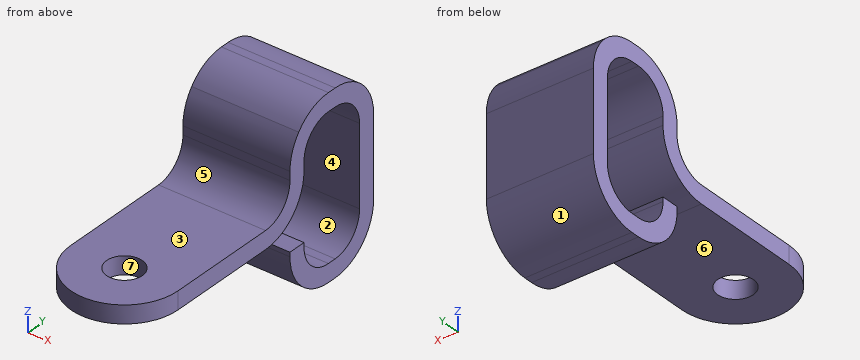
from build123d import *

# Parameters (mm, degrees)
EXTRUDE_1_DEPTH     = 1
SKETCH_2_R          = 1
CUT_EXTRUDE_1_DEPTH = 28.116287625
OTHER_START         = -3
OTHER_1_DEPTH       = 6
OTHER_1_2_DEPTH     = 6
OTHER_2_DEPTH       = 6
OTHER_2_2_DEPTH     = 6
OTHER_START_2       = -5.911973487
OTHER_2_3_OUTLINE_W = 6
OTHER_2_3_OUTLINE_H = 4
OTHER_2_3_DEPTH     = 12.911973487
OTHER_START_3       = -10.873389715
OTHER_2_4_OUTLINE_R = 1
OTHER_2_4_DEPTH     = 1
OTHER_START_4       = -8.133389715
OTHER_2_5_OUTLINE_W = 6
OTHER_2_5_OUTLINE_H = 1
OTHER_2_5_DEPTH     = 0.481416228
OTHER_2_6_DEPTH     = 6
OTHER_2_7_DEPTH     = 6


with BuildPart() as part:
    # Sketch 1 → Бобышка-Вытянуть1 (new body)
    with BuildSketch(Plane(origin=(0, 0, 0), x_dir=(1, 0, 0), z_dir=(0, 1, 0))):
        with BuildLine():
            Line((-3, 26.931265373), (-3, -3.068734627))
            ThreePointArc((-3, -3.068734627), (0, -6.068734627), (3, -3.068734627))
            Line((3, -3.068734627), (3, 26.931265373))
            Line((3, 26.931265373), (-3, 26.931265373))
        make_face()
    extrude(amount=EXTRUDE_1_DEPTH)

    # Sketch 2 → Вырез-Вытянуть1 (cut, through all)
    with BuildSketch(Plane(origin=(0, 1, 0), x_dir=(1, 0, 0), z_dir=(0, 1, 0))):
        with Locations(Location((0, -3.068734627, 0), (0, 0, 270))):
            Circle(SKETCH_2_R)
    extrude(amount=-CUT_EXTRUDE_1_DEPTH, mode=Mode.SUBTRACT)

    # Other 1: read off the stored shape, not the designer's step
    # Other 1 outline → Other 1 (cut)
    with BuildSketch(Plane.YZ.offset(OTHER_START)):
        with BuildLine():
            Line((1, -26.931265373), (1, -5.288574535))
            ThreePointArc((1, -5.288574535), (0.26258199, -4.342443478), (0, -3.171973487))
            Line((0, -3.171973487), (0, -26.931265373))
            Line((0, -26.931265373), (1, -26.931265373))
        make_face()
    extrude(amount=OTHER_1_DEPTH, mode=Mode.SUBTRACT)

    # Other 1 2 outline → Other 1 2 (add)
    with BuildSketch(Plane.YZ.offset(OTHER_START)):
        with BuildLine():
            Line((2.74, -5.911973487), (22.980708114, -5.911973487))
            Line((22.980708114, -5.911973487), (22.980708114, -4.911973487))
            Line((22.980708114, -4.911973487), (2.74, -4.911973487))
            ThreePointArc((2.74, -4.911973487), (1.509634201, -4.402339286), (1, -3.171973487))
            Line((1, -3.171973487), (1, -5.288574535))
            ThreePointArc((1, -5.288574535), (1.815848193, -5.75141983), (2.74, -5.911973487))
        make_face()
    extrude(amount=OTHER_1_2_DEPTH)

    # Other 2: read off the stored shape, not the designer's step
    # Other 2 outline → Other 2 (cut)
    with BuildSketch(Plane.YZ.offset(OTHER_START)):
        with BuildLine():
            ThreePointArc((7.221416228, -4.911973487), (8.391886219, -5.174555476), (9.338017277, -5.911973487))
            Line((9.338017277, -5.911973487), (22.980708114, -5.911973487))
            Line((22.980708114, -5.911973487), (22.980708114, -4.911973487))
            Line((22.980708114, -4.911973487), (7.221416228, -4.911973487))
        make_face()
    extrude(amount=OTHER_2_DEPTH, mode=Mode.SUBTRACT)

    # Other 2 2 outline → Other 2 2 (add)
    with BuildSketch(Plane.YZ.offset(OTHER_START)):
        with BuildLine():
            Line((8.961416228, -7.651973487), (8.961416228, -12.133389715))
            ThreePointArc((8.961416228, -12.133389715), (8.451782027, -13.363755514), (7.221416228, -13.873389715))
            Line((7.221416228, -13.873389715), (6.74, -13.873389715))
            ThreePointArc((6.74, -13.873389715), (5.509634201, -13.363755514), (5, -12.133389715))
            Line((5, -12.133389715), (5, -11.892681601))
            Line((5, -11.892681601), (4, -11.892681601))
            Line((4, -11.892681601), (4, -12.133389715))
            ThreePointArc((4, -12.133389715), (4.80252742, -14.070862295), (6.74, -14.873389715))
            Line((6.74, -14.873389715), (7.221416228, -14.873389715))
            ThreePointArc((7.221416228, -14.873389715), (9.158888808, -14.070862295), (9.961416228, -12.133389715))
            Line((9.961416228, -12.133389715), (9.961416228, -7.651973487))
            ThreePointArc((9.961416228, -7.651973487), (9.800862571, -6.72782168), (9.338017277, -5.911973487))
            Line((9.338017277, -5.911973487), (7.221416228, -5.911973487))
            ThreePointArc((7.221416228, -5.911973487), (8.451782028, -6.421607687), (8.961416228, -7.651973487))
        make_face()
    extrude(amount=OTHER_2_2_DEPTH)

    # Other 2 3 outline → Other 2 3 (cut)
    with BuildSketch(Plane.XY.offset(OTHER_START_2)):
        with Locations((0, 2)):
            Rectangle(OTHER_2_3_OUTLINE_W, OTHER_2_3_OUTLINE_H)
    extrude(amount=OTHER_2_3_DEPTH, mode=Mode.SUBTRACT)

    # Other 2 6 outline → Other 2 6 (cut)
    with BuildSketch(Plane.YZ.offset(OTHER_START)):
        with BuildLine():
            ThreePointArc((4.623398951, -5.911973487), (5.569530009, -5.174555476), (6.74, -4.911973487))
            Line((6.74, -4.911973487), (4, -4.911973487))
            Line((4, -4.911973487), (4, -5.911973487))
            Line((4, -5.911973487), (4.623398951, -5.911973487))
        make_face()
    extrude(amount=OTHER_2_6_DEPTH, mode=Mode.SUBTRACT)



with BuildPart() as body_2:
    # Other 2 4 outline → Other 2 4 (new body)
    with BuildSketch(Plane.XY.offset(OTHER_START_3)):
        with BuildLine():
            Line((3, 1), (-3, 1))
            Line((-3, 1), (-3, -3.980708114))
            ThreePointArc((-3, -3.980708114), (0, -6.980708114), (3, -3.980708114))
            Line((3, -3.980708114), (3, 1))
        make_face()
        with Locations((0, -3.980708114)):
            Circle(OTHER_2_4_OUTLINE_R, mode=Mode.SUBTRACT)
    extrude(amount=OTHER_2_4_DEPTH)


with BuildPart() as body_3:
    # Other 2 5 outline → Other 2 5 (new body)
    with BuildSketch(Plane.XY.offset(OTHER_START_4)):
        with Locations((0, 4.5)):
            Rectangle(OTHER_2_5_OUTLINE_W, OTHER_2_5_OUTLINE_H)
    extrude(amount=OTHER_2_5_DEPTH)


with BuildPart() as part_1:
    add(part.part)

    add(body_2.part)  # Other 2 7 merges body 2

    add(body_3.part)  # Other 2 7 merges body 3
    # Other 2 7 outline → Other 2 7 (add)
    with BuildSketch(Plane.YZ.offset(OTHER_START)):
        with BuildLine():
            Line((6.74, -5.911973487), (4.623398951, -5.911973487))
            ThreePointArc((4.623398951, -5.911973487), (4.160553657, -6.72782168), (4, -7.651973487))
            Line((4, -7.651973487), (5, -7.651973487))
            ThreePointArc((5, -7.651973487), (5.5096342, -6.421607687), (6.74, -5.911973487))
        make_face()
        with BuildLine():
            Line((1, -10.873389715), (2.26, -10.873389715))
            ThreePointArc((2.26, -10.873389715), (4.19747258, -10.070862295), (5, -8.133389715))
            Line((5, -8.133389715), (4, -8.133389715))
            ThreePointArc((4, -8.133389715), (3.490365799, -9.363755514), (2.26, -9.873389715))
            Line((2.26, -9.873389715), (1, -9.873389715))
            Line((1, -9.873389715), (1, -10.873389715))
        make_face()
    extrude(amount=OTHER_2_7_DEPTH)


solid = part_1.part
Geometry check sheet. Reference: the model listing, model coordinates, mm. Face numbers are marked on the shaded views. A direction names the side the tool comes from. Round coordinates to 2 decimals unless told otherwise and drop trailing zeros. Loops run counter-clockwise (first coordinate to the right, second up) from the corner with the lowest first, then second, coordinate; pieces in that order, holes last.
Item 1: Cross-section at C-C on z = -13. Record the boundary of the cut face in (x, y), then the cut area to 3 significant figures.
Item 2: Cross-section at B-B on y = -4.75. Record the boundary of the cut face in (x, z).
Item 3: Thickness scan on line 1 (Z direction, x = 0.65, y = 6.75); line 2 (Y direction, x = -1.4, z = -12.25); line 3 (Y direction, x = 0, z = -10.4). Record the ranges inside material, lowest first.
Item 4: Gauge pin test, flat ends, axial feed: pin 1 (2.5 mm diameter, centred on x = 0, y = -3.98, fed in from +Z); pin 2 (0.5 mm diameter, centred on x = 0.5, y = 4.5, fed in from +Z); pin 3 (0.5 mm diameter, centred on x = -1, z = -8, fed in from -Y). Record the tip position at first contact, or that the pin passes through.
Item 5: Access from +Z, -Z, +X, -X, +Y, -Y to the whole of each face (thin tool, end or side, straight path). Record for the marked faces 1, 2 and 3.
Item 6: Cross-section at D-D on x = -1.7. Record the boundary of the cut face in (y, z).
Item 7: Mould release check, pull along Z, two halves, no side actions. Record for the marked faces 4, 5, 6 and 7: pulls with the +Z half, pulls with the -Z half, needs draft (parallel to the pull), parting line crosses it, or undercut.
Item 8: Cross-section at A-A on x = 0. Record the boundary of the cut face in (y, z).
Answer sheet:
1. outline: (-3, 4.14) - (3, 4.14) - (3, 5.23) - (-3, 5.23) - close; (-3, 8.73) - (3, 8.73) - (3, 9.82) - (-3, 9.82) - close
1. area: 13.1 mm2
2. outline: (-2.9, -10.87) - (-0.64, -10.87) - (-0.64, -9.87) - (-2.9, -9.87) - close; (0.64, -10.87) - (2.9, -10.87) - (2.9, -9.87) - (0.64, -9.87) - close
3. line 1: z = -14.87 to -13.87, -5.91 to -4.91
3. line 2: y = 4 to 5, 8.96 to 9.96
3. line 3: y = -6.98 to -4.98, -2.98 to 3.8, 8.96 to 9.96
4. pin 1: stops at z = -9.87
4. pin 2: stops at z = -5.77
4. pin 3: stops at y = 4
5. face 1: -Z, +X, -X, +Y
5. face 2: +X, -X
5. face 3: +Z, +X, -X, -Y
6. outline: (-6.45, -10.87) - (2.26, -10.87) arc R2.74 ccw to (5, -8.13) - (5, -7.65) arc R1.74 cw to (6.74, -5.91) - (7.22, -5.91) arc R1.74 cw to (8.96, -7.65) - (8.96, -12.13) arc R1.74 cw to (7.22, -13.87) - (6.74, -13.87) arc R1.74 cw to (5, -12.13) - (5, -11.89) - (4, -11.89) - (4, -12.13) arc R2.74 ccw to (6.74, -14.87) - (7.22, -14.87) arc R2.74 ccw to (9.96, -12.13) - (9.96, -7.65) arc R2.74 ccw to (7.22, -4.91) - (6.74, -4.91) arc R2.74 ccw to (4, -7.65) - (4, -8.13) arc R1.74 cw to (2.26, -9.87) - (-6.45, -9.87) - close
7. face 4: undercut
7. face 5: pulls with the +Z half
7. face 6: pulls with the -Z half
7. face 7: needs draft
8. outline: (-6.98, -10.87) - (-4.98, -10.87) - (-4.98, -9.87) - (-6.98, -9.87) - close; (-2.98, -10.87) - (2.26, -10.87) arc R2.74 ccw to (5, -8.13) - (5, -7.65) arc R1.74 cw to (6.74, -5.91) - (7.22, -5.91) arc R1.74 cw to (8.96, -7.65) - (8.96, -12.13) arc R1.74 cw to (7.22, -13.87) - (6.74, -13.87) arc R1.74 cw to (5, -12.13) - (5, -11.89) - (4, -11.89) - (4, -12.13) arc R2.74 ccw to (6.74, -14.87) - (7.22, -14.87) arc R2.74 ccw to (9.96, -12.13) - (9.96, -7.65) arc R2.74 ccw to (7.22, -4.91) - (6.74, -4.91) arc R2.74 ccw to (4, -7.65) - (4, -8.13) arc R1.74 cw to (2.26, -9.87) - (-2.98, -9.87) - close
